from build123d import *

# Parameters (mm, degrees)
SKETCH_1_W          = 10
SKETCH_1_H          = 20
SKETCH_1_W_2        = 7.6
SKETCH_1_H_2        = 17.6
EXTRUDE_1_DEPTH     = 145
SKETCH_3_R          = 2.15
CUT_EXTRUDE_1_DEPTH = 147.458185159
SKETCH_4_R          = 2.15
CUT_EXTRUDE_2_DEPTH = 146.688022843


with BuildPart() as part:
    # ｽｹｯﾁ1 → 押し出し-薄板1 (new body)
    with BuildSketch(Plane(origin=(0, 0, 0), x_dir=(0, 0, -1), z_dir=(1, 0, 0))):
        Rectangle(SKETCH_1_W, SKETCH_1_H)
        Rectangle(SKETCH_1_W_2, SKETCH_1_H_2, mode=Mode.SUBTRACT)
    extrude(amount=EXTRUDE_1_DEPTH)

    # ｽｹｯﾁ3 → ｶｯﾄ - 押し出し1 (cut, through all)
    with BuildSketch(Plane(origin=(0, 10, 0), x_dir=(1, 0, 0), z_dir=(0, 1, 0))):
        with Locations(Location((92.5, 0, 0), (0, 0, 270))):
            Circle(SKETCH_3_R)
        with Locations(Location((52.5, 0, 0), (0, 0, 270))):
            Circle(SKETCH_3_R)
        with Locations(Location((72.5, 0, 0), (0, 0, 270))):
            Circle(SKETCH_3_R)
    extrude(amount=-CUT_EXTRUDE_1_DEPTH, mode=Mode.SUBTRACT)

    # ｽｹｯﾁ4 → ｶｯﾄ - 押し出し2 (cut, through all)
    with BuildSketch(Plane.XY.offset(5)):
        with Locations((140, 5)):
            Circle(SKETCH_4_R)
        with Locations(Location((140, -5, 0), (0, 0, 90))):
            Circle(SKETCH_4_R)
        with Locations(Location((5, 5, 0), (0, 0, 90))):
            Circle(SKETCH_4_R)
        with Locations((5, -5)):
            Circle(SKETCH_4_R)
    extrude(amount=-CUT_EXTRUDE_2_DEPTH, mode=Mode.SUBTRACT)


solid = part.part
Here's how the part is built. I have some questions about the finished solid (model axes, mm). A direction names the side the tool comes from. Coordinates: 2 decimals unless noted, no trailing zeros. Order: outer loops, then holes, each group sorted by start corner. A loop starts at its lowest first (then second) coordinate and runs counter-clockwise, first axis right, second up.
Item 1: If we section it at B-B on y = 5: List the corners of the cut face in (x, z) for me.
Result sheet:
outline: (0, -5) - (2.85, -5) - (2.85, -3.8) - (0, -3.8) - close; (0, 3.8) - (2.85, 3.8) - (2.85, 5) - (0, 5) - close; (7.15, -5) - (137.85, -5) - (137.85, -3.8) - (7.15, -3.8) - close; (7.15, 3.8) - (137.85, 3.8) - (137.85, 5) - (7.15, 5) - close; (142.15, -5) - (145, -5) - (145, -3.8) - (142.15, -3.8) - close; (142.15, 3.8) - (145, 3.8) - (145, 5) - (142.15, 5) - close
Item 2: If we section it at D-D on x = 72.5: List the corners of the cut face in (y, z) for me.
Result sheet:
outline: (-10, -5) - (10, -5) - (10, -2.15) - (8.8, -2.15) - (8.8, -3.8) - (-8.8, -3.8) - (-8.8, -2.15) - (-10, -2.15) - close; (-10, 2.15) - (-8.8, 2.15) - (-8.8, 3.8) - (8.8, 3.8) - (8.8, 2.15) - (10, 2.15) - (10, 5) - (-10, 5) - close
Item 3: If we section it at C-C on z = 0: State how many separate pieces and enclosed holes the cut face has, plus the area to 3 significant figures.
Result sheet:
separate pieces: 8
enclosed holes: 0
area: 317 mm2
Item 4: For faces 1 (the face through (90.4, 9.41, -0.47)), 2 (the face through (71, -8.8, 3)), which set-ups out of +Z, -Z, +X, -X, +Y, -Y let a thin tool reach every point of the face, with its end or its side?
Result sheet:
face 1: +Y, -Y
face 2: +X, -X
Item 5: I need wall thicknesses on line 1 (X direction, y = 9.25, z = 0); line 2 (Z direction, x = 86, y = 2.5); line 3 (Y direction, x = 28, z = -1.5). Which ranges of each line are inside material? Lowest first, please.
Result sheet:
line 1: x = 0 to 50.35, 54.65 to 70.35, 74.65 to 90.35, 94.65 to 145
line 2: z = -5 to -3.8, 3.8 to 5
line 3: y = -10 to -8.8, 8.8 to 10
Item 6: If we section it at A-A on x = 129.5: List the corners of the cut face in (y, z) for me.
Result sheet:
outline: (-10, -5) - (10, -5) - (10, 5) - (-10, 5) - close; hole (-8.8, -3.8) - (8.8, -3.8) - (8.8, 3.8) - (-8.8, 3.8) - close
Item 7: If we mould it in two halves opening along Y, with no side actions, what happens to faces 3 (the face through (54.31, -9.39, 1.16)), 4 (the face through (3.294, -6.308, -4.392)), 5 (the face through (71, 10, -2))? For each: +Y half, -Y half, draft (parallel to the pull), parting line (faces both ways), or undercut.
Result sheet:
face 3: draft
face 4: undercut
face 5: +Y half
